Check sheet for the modelled part. Datum: model origin and axes. Units: mm. Face numbers are marked on the shaded views. A direction names the side the tool comes from. Coordinates: 2 decimals unless noted, no trailing zeros. Write each loop counter-clockwise with the first axis right and the second up, starting at its lowest first coordinate (ties: lowest second). Pieces come first, ordered by that corner, then holes. Notation, with made-up numbers: (-30, 85.5) -> (8, 85.5) arc R14 ccw to (8, 110.5) -> close; hole circle Ø10 at (1.25, -20). An arc over 180 degrees is marked (long way). Put each result on its own line as item: value.
```python
from build123d import *

# Parameters (mm, degrees)
KREISMUSTER1_COUNT = 3
VERRUNDUNG1_R      = 1


with BuildPart() as part:
    # Skizze2 → Rotation1 (revolve)
    with BuildSketch(Plane(origin=(0, 0, 0), x_dir=(0, 0, -1), z_dir=(1, 0, 0)), mode=Mode.PRIVATE) as rotation1_sk:
        Polygon((9.5, 7), (8.5, 7), (8.5, 25), (2.5, 25), (2.5, 7.5), (7, 7.5), (7, 6), (7.5, 6), (7.5, 4), (18.5, 4), (18.5, 5), (9.5, 5), align=None)
    revolve(rotation1_sk.sketch.rotate(Axis((0, 0, 0), (0, 0, -1)), 90), axis=Axis((0, 0, 0), (0, 0, -1)))

    # Skizze4 → Ø7.1 (7.1) Durchmesser Bohrung1 (revolve, cut)
    with BuildSketch(Plane(origin=(0, 15, -2.5), x_dir=(0, -1, 0), z_dir=(1, 0, 0))):
        Polygon((0, 0), (0, 11.633055198), (3.55, 9.5), (3.55, 0), align=None)
    f_7_1_7_1_durchmesser_bohrung1 = revolve(axis=Axis((0, 15, 3.85), (0, 0, -1)), mode=Mode.SUBTRACT)

    # Kreismuster1: Ø7.1 (7.1) Durchmesser Bohrung1 ×3 about axis
    kreismuster1_axis = Axis((0, 0, 0), (0, 0, 1))
    for i in range(1, KREISMUSTER1_COUNT):
        add(f_7_1_7_1_durchmesser_bohrung1.rotate(kreismuster1_axis, i * 360 / KREISMUSTER1_COUNT), mode=Mode.SUBTRACT)

    # Verrundung1
    verrundung1_edges = [part.edges().sort_by_distance(p)[0] for p in [
        (-25, 0, -8.5),
        (-7.5, 0, -2.5),
        (-5, 0, -18.5),
    ]]
    fillet(verrundung1_edges, radius=VERRUNDUNG1_R - 0.0001)  # a hair under: the kernel refuses the full size


solid = part.part
```
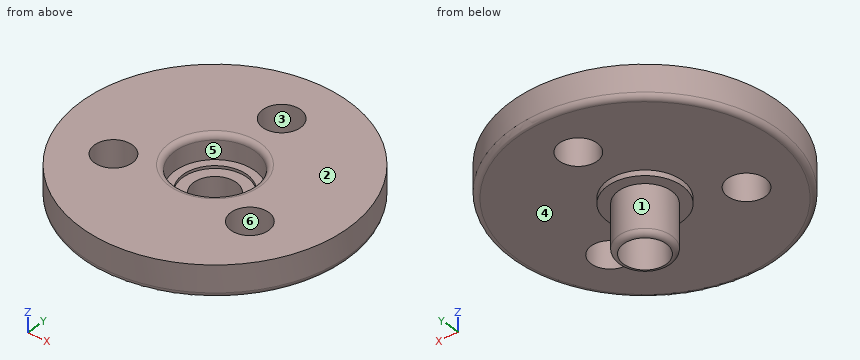
Q1. Mould release check, pull along Y, two halves, no side actions. Record for the marked faces 1, 2 and 3: released by +Y, released by -Y, zero draft, split by the parting line, or undercut.
Recorded:
face 1: split by the parting line
face 2: zero draft
face 3: undercut
Q2. Tool access check on the marked faces 4, 5 and 6. Record the directions out of +Z, -Z, +X, -X, +Y, -Y that give a thin tool (end or side, any length) a straight path to the whole face; none if there is none.
Recorded:
face 4: -Z
face 5: +Z
face 6: +Z, -Z
Q3. Cross-section at A-A (x = 0). State how many separate pieces and enclosed holes the cut face has, plus the area to 3 significant figures.
Recorded:
separate pieces: 3
enclosed holes: 0
area: 199 mm2
Q4. Cross-section at D-D (z = -5.75). Record the cut outline in (x, y) (3 decimals).
Recorded:
outline: circle Ø50 at (0, 0); hole circle Ø7.1 at (-12.99, -7.5); hole circle Ø15 at (0, 0); hole circle Ø7.1 at (0, 15); hole circle Ø7.1 at (12.99, -7.5)
Q5. Material ranges on line 1 along Y through (x, z) = (0, -6.25); line 2 along Y through (x, z) = (0, -14); line 3 along Z through (x, y) = (10, 6), recorded low to high.
Recorded:
line 1: y = -25 to -7.5, 7.5 to 11.45, 18.55 to 25
line 2: y = -5 to -4, 4 to 5
line 3: z = -8.5 to -2.5
Q6. Cross-section at C-C (z = -11.75). Record the cut outline in (x, y), plus the area to 3 significant figures.
Recorded:
outline: circle Ø10 at (0, 0); hole circle Ø8 at (0, 0)
area: 28.3 mm2
Q7. Depth check by flat-ended pin: P1, Ø8, axis at x = -12.99, y = -7.5, coming from the -Z side; P2, Ø5, axis at x = -7, z = -8.5, coming from the -Y side; P3, Ø9.5, axis at x = -2, y = 2.5, coming from the +Z side. Enter the tip coordinate at first touch or a pass-through.
Recorded:
P1: stops at z = -8.5
P2: stops at y = -24.56
P3: stops at z = -2.66
